Verification items for this drawing (mm, ordinates from the low corner). Give positions to 0.01 mm unless a question says otherwise; leave off trailing zeros. Write each loop counter-clockwise with the first axis right and the second up, starting at its lowest first coordinate (ties: lowest second). Pieces come first, ordered by that corner, then holes. Notation, with made-up numbers: (-11.5, -14) -> (37.5, -14) arc R7 ccw to (37.5, -5) -> close; hole circle Ø9 at (75, 0.25). An arc over 180 degrees is marked (long way). Answer as a JSON object with one key per item and string values.
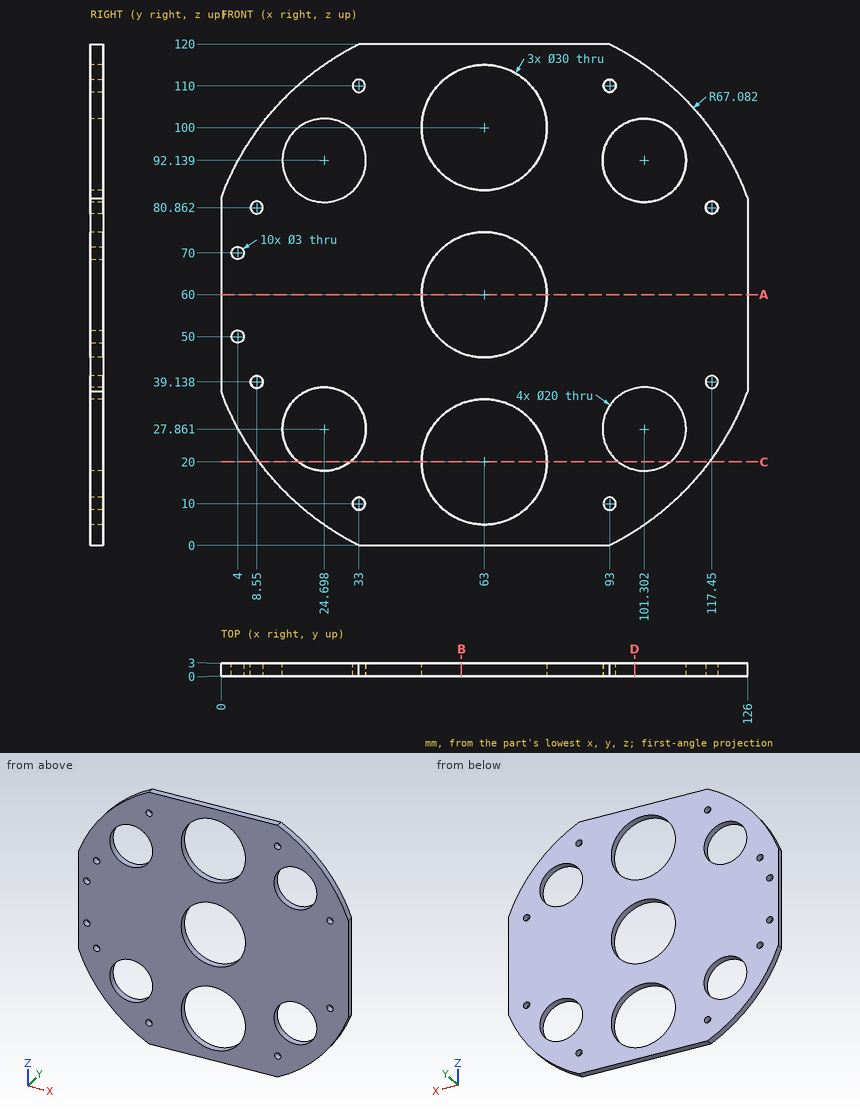
1. Go/stop test with a flat-tipped pin: P1, Ø2.5, axis at x = 33, z = 110, coming from the +Y side. Record where the tip stops, or that it passes through.
Determined:
{"P1": "through"}
2. Sectioned sample at D-D, the plane x = 99. Enter the section's corners in (y, z), plus the area to 3 significant figures.
Determined:
{"outline": "(0, 3.4) -> (3, 3.4) -> (3, 18.13) -> (0, 18.13) -> close; (0, 37.59) -> (3, 37.59) -> (3, 82.41) -> (0, 82.41) -> close; (0, 101.87) -> (3, 101.87) -> (3, 116.6) -> (0, 116.6) -> close", "area": "223 mm^2"}
3. Sectioned sample at A-A, the plane z = 60. Enter the section's corners in (x, y).
Determined:
{"outline": "(0, 0) -> (48, 0) -> (48, 3) -> (0, 3) -> close; (78, 0) -> (126, 0) -> (126, 3) -> (78, 3) -> close"}
4. Scan lines: L1, parallel to X at y = 2.7, z = 38 (1 decimal); L2, parallel to Z at x = 75, y = 1; L3, parallel to Z at x = 98, y = 2.45. Record each from-to range of solid material in increasing order. Write a range as [from, to].
Determined:
{"L1": "[0, 7.6], [9.5, 116.5], [118.4, 126]", "L2": "[0, 11], [29, 51], [69, 91], [109, 120]", "L3": "[2.77, 18.42], [37.3, 82.7], [101.58, 117.23]"}
5. Sectioned sample at C-C, the plane z = 20. Enter the section's corners in (x, y), plus the area to 3 significant figures.
Determined:
{"outline": "(9.15, 0) -> (18.52, 0) -> (18.52, 3) -> (9.15, 3) -> close; (30.88, 0) -> (48, 0) -> (48, 3) -> (30.88, 3) -> close; (78, 0) -> (95.12, 0) -> (95.12, 3) -> (78, 3) -> close; (107.48, 0) -> (116.85, 0) -> (116.85, 3) -> (107.48, 3) -> close", "area": "159 mm^2"}
6. Sectioned sample at B-B, the plane x = 57.5. Enter the section's corners in (y, z) (1 decimal), plus the area to 3 significant figures.
Determined:
{"outline": "(0, 0) -> (3, 0) -> (3, 6) -> (0, 6) -> close; (0, 34) -> (3, 34) -> (3, 46) -> (0, 46) -> close; (0, 74) -> (3, 74) -> (3, 86) -> (0, 86) -> close; (0, 114) -> (3, 114) -> (3, 120) -> (0, 120) -> close", "area": "109 mm^2"}
